The model under review builds one solid part; all positions refer to its coordinate system, in mm. A direction names the side the tool comes from. Round coordinates to 2 decimals unless told otherwise and drop trailing zeros. Loops run counter-clockwise (first coordinate to the right, second up) from the corner with the lowest first, then second, coordinate; pieces in that order, holes last. Notation, with made-up numbers: (0, 40.25) -> (57, 40.25) arc R28 ccw to (57, 61.25) -> close; hole circle Ø11 at (87, 3). An arc over 180 degrees is marked (long way). Return JSON: item names as keys, results as strings. Group by question number.
```python
from build123d import *

# Parameters (mm, degrees)
F0_R     = 25.4
F1_DEPTH = 25.4
F2_R     = 5.08


with BuildPart() as f1:
    # F0 (on Front) → F1 (new body)
    with BuildSketch(Plane.XZ):
        Circle(F0_R)
        with BuildLine():
            ThreePointArc((1.27, 6.221704), (0, -6.35), (-1.27, 6.221704))
            Line((-1.27, 6.221704), (-1.27, 8.351671))
            Line((-1.27, 8.351671), (1.27, 8.351671))
            Line((1.27, 8.351671), (1.27, 6.221704))
        make_face(mode=Mode.SUBTRACT)
    extrude(amount=F1_DEPTH)

    # F2
    f2_edges = [f1.edges().sort_by_distance(p)[0] for p in [
        (-25.4, 0, 0),
        (-25.4, -25.4, 0),
    ]]
    fillet(f2_edges, radius=F2_R)


solid = f1.part
```
1. We need section D-D, the plane y = -23.25. Write out the cut boundary in (x, z), then the cut area to 3 significant figures.
2. We need section B-B, the plane z = 0. Write out the cut boundary in (x, y).
3. Tool access review of faces 4 (the face through (-5, -25.4, 5)), 5 (the face through (-1.27, -13, 7)): name each direction out of +Z, -Z, +X, -X, +Y, -Y from which nothing blocks a thin tool from reaching the whole face with its end or side.
4. For P1, Ø6, axis at x = -1.5, z = 1, coming from the -Y side; P2, Ø2.5, axis at y = -17.5, z = 7.5, coming from the -X side; P3, Ø8, axis at y = -17.5, z = -20.5, coming from the -X side; P4, Ø3, axis at x = -0.5, y = -11, coming from the -Z side, all flat-tipped, find the tip position at first contact; note any pin that passes through.
5. We need section C-C, the plane y = -14. Write out the cut boundary in (x, z), then the cut area to 3 significant figures.
6. Draft analysis for pull direction X (two halves, no side actions). For faces 1 (the face through (-5.506, -12.593, -24.796)), 2 (the face through (1.27, -13, 7)), 3 (the face through (-5, 0, 5)), state which applies: pulls with the +X half, pulls with the -X half, needs draft (parallel to the pull), parting line crosses it, or undercut.
7. We need section A-A, the plane x = 0. Write out the cut boundary in (y, z).
8. Wall thickness on line 1 (Z direction, x = 0, y = -16); line 2 (X direction, y = -0.75, z = -5.5); line 3 (Z direction, x = -3, y = -14.5): over which ranges is each line inside the solid? List them lowest first.
Check sheet entries:
{
 "1": {"outline": "circle Ø48.94 at (0, 0); hole (-1.27, 6.22) arc R6.35 ccw (long way) to (1.27, 6.22) -> (1.27, 8.35) -> (-1.27, 8.35) -> close", "area": "1,750 mm²"},
 "2": {"outline": "(-25.4, -20.32) arc R5.08 ccw to (-20.32, -25.4) -> (-6.35, -25.4) -> (-6.35, 0) -> (-20.32, 0) arc R5.08 ccw to (-25.4, -5.08) -> close; (6.35, -25.4) -> (20.32, -25.4) arc R5.08 ccw to (25.4, -20.32) -> (25.4, -5.08) arc R5.08 ccw to (20.32, 0) -> (6.35, 0) -> close"},
 "3": {"face 4": "+Z, -Z, +X, -X, -Y", "face 5": "+Y, -Y"},
 "4": {"P1": "passes through", "P2": "stops at x = -24.62", "P3": "stops at x = -19.31", "P4": "stops at z = -25.4"},
 "5": {"outline": "circle Ø50.8 at (0, 0); hole (-1.27, 6.22) arc R6.35 ccw (long way) to (1.27, 6.22) -> (1.27, 8.35) -> (-1.27, 8.35) -> close", "area": "1,890 mm²"},
 "6": {"face 1": "parting line crosses it", "face 2": "undercut", "face 3": "needs draft"},
 "7": {"outline": "(-25.4, -20.32) arc R5.08 ccw to (-20.32, -25.4) -> (-5.08, -25.4) arc R5.08 ccw to (0, -20.32) -> (0, -6.35) -> (-25.4, -6.35) -> close; (-25.4, 8.35) -> (0, 8.35) -> (0, 20.32) arc R5.08 ccw to (-5.08, 25.4) -> (-20.32, 25.4) arc R5.08 ccw to (-25.4, 20.32) -> close"},
 "8": {"line 1": "z = -25.4 to -6.35, 8.35 to 25.4", "line 2": "x = -22.31 to -3.17, 3.17 to 22.31", "line 3": "z = -25.22 to -5.6, 5.6 to 25.22"}
}
